Autodesk Fusion 360 part; units mm, degrees
sketch "Sketch1" plane through (0, 0, 0) normal (0, 0, 1) x (1, 0, 0)
  line L0 (0, 0) -> (0, 30)
  line L1 (0, 30) -> (30, 30)
  line L2 (30, 30) -> (30, 20)
  line L3 (30, 20) -> (50, 20)
  line L4 (50, 20) -> (50, 30)
  line L5 (50, 30) -> (80, 30)
  line L6 (80, 30) -> (100, 10)
  line L7 (100, 10) -> (100, 0)
  line L8 (100, 0) -> (0, 0)
revolve "Revolve1" add sketch "Sketch1" angle 360 about axis through (100, 0, 0) along (-1, 0, 0)
Design review of the part built by this model. Coordinates are the model's own, in mm. A direction names the side the tool comes from. Round coordinates to 2 decimals unless told otherwise and drop trailing zeros. Write each loop counter-clockwise with the first axis right and the second up, starting at its lowest first coordinate (ties: lowest second). Pieces come first, ordered by that corner, then holes. Notation, with made-up numbers: (-16, 36.5) -> (12, 36.5) arc R27 cw to (12, 62.5) -> close; hole circle Ø5 at (-20.75, -18). An arc over 180 degrees is marked (long way). Answer in a Markdown table with one row per item.
Q1. For faces 1 (the face through (30, 6, 20)), 2 (the face through (15.21, -29.97, 1.32)), list the 3-axis set-ups (+Z, -Z, +X, -X, +Y, -Y) from which the entire face can be reached by the end or side of a thin tool; tool diameter is ignored.
The answers:
| item | result |
|---|---|
| face 1 | none |
| face 2 | +X, -X |
Q2. Draft analysis for pull direction X (two halves, no side actions). For faces 3 (the face through (40.14, -4.336, -19.524)), 4 (the face through (100, 0, 0)), 5 (the face through (0, 0, 0)), 6 (the face through (65.21, -29.97, 1.32)), state which applies: +X half, -X half, draft (parallel to the pull), parting line (faces both ways), or undercut.
The answers:
| item | result |
|---|---|
| face 3 | undercut |
| face 4 | +X half |
| face 5 | -X half |
| face 6 | draft |
Q3. Take a section at A-A, the plane y = 0. State the section outline as (x, z) points, then the cut area to 3 significant figures.
The answers:
| item | result |
|---|---|
| outline | (0, -30) -> (30, -30) -> (30, -20) -> (50, -20) -> (50, -30) -> (80, -30) -> (100, -10) -> (100, 10) -> (80, 30) -> (50, 30) -> (50, 20) -> (30, 20) -> (30, 30) -> (0, 30) -> close |
| area | 5,200 mm² |
Q4. To check wall thickness, follow L1, parallel to X at y = 21, z = -20; L2, parallel to X at y = -24, z = -5.5; L3, parallel to Y at x = 29, z = 12. State the ranges of each line that lie inside material, in increasing order. Write a range as [from, to].
The answers:
| item | result |
|---|---|
| L1 | [0, 30], [50, 81] |
| L2 | [0, 30], [50, 85.38] |
| L3 | [-27.5, 27.5] |
Q5. Take a section at C-C, the plane x = 84. State the section outline as (y, z) points, then the cut area to 3 significant figures.
The answers:
| item | result |
|---|---|
| outline | circle Ø52 at (0, 0) |
| area | 2,120 mm² |
Q6. Take a section at D-D, the plane x = 7.5. State the section outline as (y, z) points, then the cut area to 3 significant figures.
The answers:
| item | result |
|---|---|
| outline | circle Ø60 at (0, 0) |
| area | 2,830 mm² |
Q7. Clearance check with flat-ended pins moving along their axes: pin 1 Ø10 at (x, z) = (61, -15) entering from -Y; pin 2 Ø8 at (y, z) = (15.5, 15) entering from +X; pin 3 Ø12 at (x, z) = (66.5, 9) entering from -Y. State where each tip first meets the part, or that it passes through.
The answers:
| item | result |
|---|---|
| pin 1 | y = -28.28 |
| pin 2 | x = 92.43 |
| pin 3 | y = -29.85 |
